Geometry check sheet. Reference: drawing and pictorial views, mm from the part's lowest x, y, z. A direction names the side the tool comes from. Round coordinates to 2 decimals unless told otherwise and drop trailing zeros. Loops run counter-clockwise (first coordinate to the right, second up) from the corner with the lowest first, then second, coordinate; pieces in that order, holes last. Notation, with made-up numbers: (-28, 12) - (19, 12) arc R21 ccw to (19, 29) - close; hole circle Ø3 at (49.25, 64.5). An arc over 180 degrees is marked (long way). Answer as CSV lines item,"result". Start each with the question number.
1) Thickness scan on line 1 along Z through (x, y) = (26.25, 18); line 2 along X through (y, z) = (15.75, 10.75); line 3 along X through (y, z) = (17.75, 11.25). Record the ranges inside material, lowest first.
2) Draft check along Z on the marked faces 5, 6, 7 and 8. Enter one of: released by +Z, released by -Z, zero draft, split by the parting line, or undercut.
3) Cross-section at A-A on y = 24.5. Record the boundary of the cut face in (x, z).
4) Cross-section at C-C on z = 22.5. Record the boundary of the cut face in (x, y) (1 decimal), and give its area (3 significant figures).
5) Depth check by flat-ended pin: P1, Ø1.2, axis at x = 36.5, y = 17.5, coming from the +Z side; P2, Ø3, axis at y = 5.5, z = 10.5, coming from the -X side; P3, Ø7.5, axis at y = 12.5, z = 8.5, coming from the +X side. Enter the tip coordinate at first touch or a pass-through.
6) Cross-section at D-D on x = 54. Record the boundary of the cut face in (y, z).
7) Access from +Z, -Z, +X, -X, +Y, -Y to the whole of each face (thin tool, end or side, straight path). Record for the marked faces 1, 2, 3 and 4.
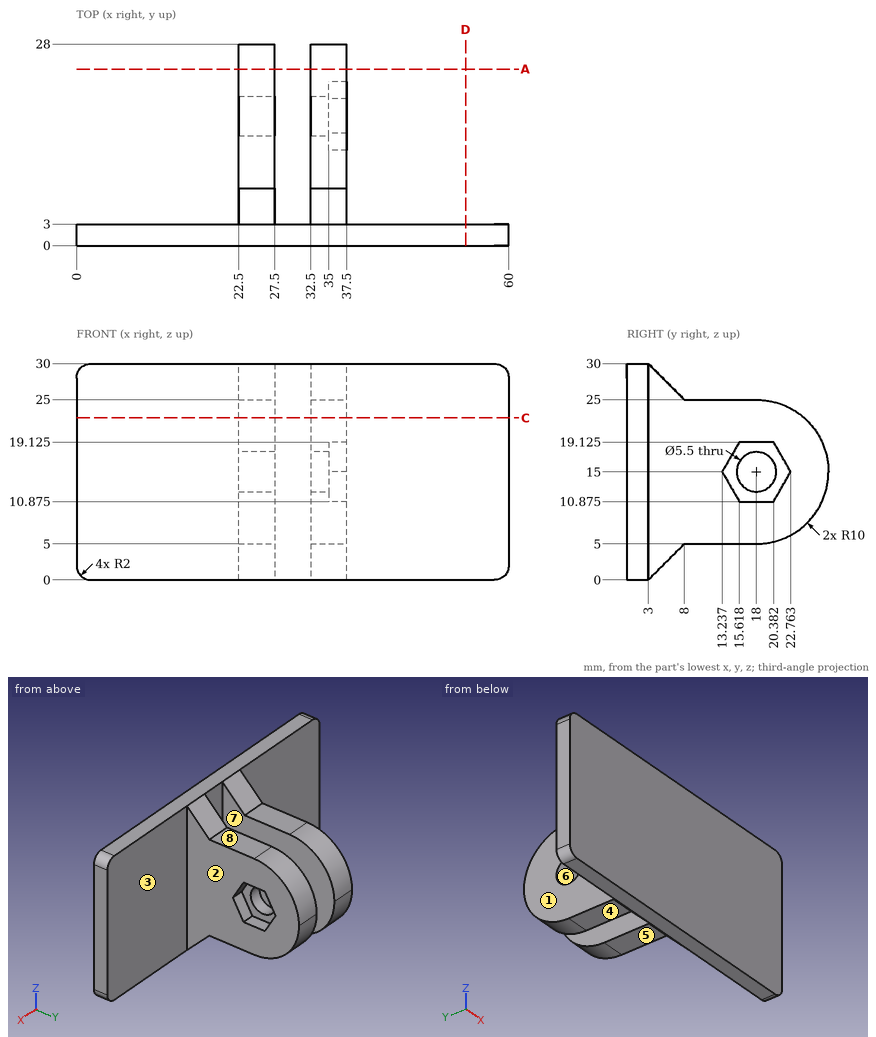
Answer block:
1,line 1,"z = 5 to 12.25, 17.75 to 25"
1,line 2,"x = 22.5 to 27.5, 32.5 to 37.5"
1,line 3,"x = 22.5 to 27.5, 32.5 to 35"
2,face 5,"released by -Z"
2,face 6,"undercut"
2,face 7,"zero draft"
2,face 8,"released by +Z"
3,outline,"(22.5, 7.4) - (27.5, 7.4) - (27.5, 22.6) - (22.5, 22.6) - close; (32.5, 7.4) - (37.5, 7.4) - (37.5, 22.6) - (32.5, 22.6) - close"
4,outline,"(0, 0) - (60, 0) - (60, 3) - (37.5, 3) - (37.5, 24.6) - (32.5, 24.6) - (32.5, 3) - (27.5, 3) - (27.5, 24.6) - (22.5, 24.6) - (22.5, 3) - (0, 3) - close"
4,area,"396 mm^2"
5,P1,"stops at z = 25"
5,P2,"stops at x = 22.5"
5,P3,"stops at x = 37.5"
6,outline,"(0, 0) - (3, 0) - (3, 30) - (0, 30) - close"
7,face 1,"+Z, -Z, -X, +Y"
7,face 2,"+Z, -Z, +X, +Y"
7,face 3,"+Z, -Z, +X, +Y"
7,face 4,"-Z, +X, -X, +Y"
